from build123d import *

# Parameters (mm, degrees)
SKETCH_1_W          = 7.5
SKETCH_1_H          = 6
EXTRUDE_1_DEPTH     = 2
SKETCH_2_W          = 12.9
SKETCH_2_H          = 3.9
EXTRUDE_2_DEPTH     = 52
SKETCH_3_R          = 1.6
CUT_EXTRUDE_1_DEPTH = 356
SKETCH_4_W          = 7.5
SKETCH_4_H          = 1.05
CUT_EXTRUDE_2_DEPTH = 10


with BuildPart() as part:
    # 草图1 → 凸台-拉伸1 (new body)
    with BuildSketch(Plane.XY):
        with Locations((3.75, 0)):
            Rectangle(SKETCH_1_W, SKETCH_1_H)
    extrude(amount=EXTRUDE_1_DEPTH)

    # 草图2 → 凸台-拉伸2 (add)
    with BuildSketch(Plane.XY.offset(2)):
        Rectangle(SKETCH_2_W, SKETCH_2_H)
    extrude(amount=EXTRUDE_2_DEPTH)

    # 草图3 → 切除-拉伸1 (cut)
    with BuildSketch(Plane.XZ.offset(1.95)):
        with Locations((3.5, 37)):
            Circle(SKETCH_3_R)
        with Locations((3.5, 11)):
            Circle(SKETCH_3_R)
        with Locations((-3.5, 24)):
            Circle(SKETCH_3_R)
        with Locations((0, 50)):
            Circle(SKETCH_3_R)
    extrude(amount=-CUT_EXTRUDE_1_DEPTH, mode=Mode.SUBTRACT)

    # 草图4 → 切除-拉伸2 (cut)
    with BuildSketch(Plane.XY.offset(2)):
        with Locations((3.75, 2.475)):
            Rectangle(SKETCH_4_W, SKETCH_4_H)
    extrude(amount=-CUT_EXTRUDE_2_DEPTH, mode=Mode.SUBTRACT)


solid = part.part
The listing builds one solid part. Answer for the finished solid, in the listing's coordinates (mm). A direction names the side the tool comes from. Round coordinates to 2 decimals unless told otherwise and drop trailing zeros. Order: outer loops, then holes, each group sorted by start corner. A loop starts at its lowest first (then second) coordinate and runs counter-clockwise, first axis right, second up. Notation, with made-up numbers: (24, 67) -> (77, 67) arc R19 ccw to (77, 84) -> close; hole circle Ø6 at (4.5, -18.5). An arc over 180 degrees is marked (long way). Put each result on its own line as item: value.
Q1. Which of the six approach directions +Z, -Z, +X, -X, +Y, -Y give full straight-line access (tool end or side, diameter ignored) to faces 1 (the flat face through (-6.45, 0, 28)), 2 (the flat face through (6.45, 0, 28)), 3 (the flat face through (0, 0, 54)), 4 (the flat face through (-3, 0, 2)), 5 (the flat face through (0, -1.95, 28))?
Results list:
face 1: +Z, -Z, -X, +Y, -Y
face 2: +Z, +X, +Y, -Y
face 3: +Z, +X, -X, +Y, -Y
face 4: -Z, -X, +Y, -Y
face 5: +Z, +X, -X, -Y
Q2. Consider line 1 along Z through (x, y) = (3.5, -1.05); line 2 along Z through (x, y) = (4.25, -1.55); line 3 along Z through (x, y) = (-3.5, 0.2). Determine where each line is inside the solid, lowest interval first.
Results list:
line 1: 0 to 9.4, 12.6 to 35.4, 38.6 to 54
line 2: 0 to 9.59, 12.41 to 35.59, 38.41 to 54
line 3: 2 to 22.4, 25.6 to 54
Q3. Section B-B, the plane x = -2.5 is taken. Write down the section's boundary in (y, z).
Results list:
outline: (-1.95, 2) -> (1.95, 2) -> (1.95, 22.75) -> (-1.95, 22.75) -> close; (-1.95, 25.25) -> (1.95, 25.25) -> (1.95, 54) -> (-1.95, 54) -> close
Q4. Each of these flat-tipped pins is pushed along its axis until it touches: P1, Ø1, axis at x = -1.5, z = 37, coming from the -Y side; P2, Ø1, axis at y = -1.5, z = 1, coming from the -X side; P3, Ø1.2, axis at y = 0.5, z = 26, coming from the +X side. Where does it stop, or does it pass through?
Results list:
P1: y = -1.95
P2: x = 0
P3: x = 6.45
Q5. Determine the mould class of faces 6 (the flat face through (5.1, -2.2, 2)), 7 (the cylindrical face through (-3.708, -0.027, 25.586)), 8 (the flat face through (7.5, -1, 1)), 9 (the cylindrical face through (4.24, -0.03, 35.58)) for opening direction X: pulls with the +X half, pulls with the -X half, needs draft (parallel to the pull), parting line crosses it, or undercut.
Results list:
face 6: needs draft
face 7: undercut
face 8: pulls with the +X half
face 9: undercut
Q6. Section D-D, the plane x = 3.5 is taken. Write down the section's boundary in (y, z).
Results list:
outline: (-3, 0) -> (1.95, 0) -> (1.95, 9.4) -> (-1.95, 9.4) -> (-1.95, 2) -> (-3, 2) -> close; (-1.95, 12.6) -> (1.95, 12.6) -> (1.95, 35.4) -> (-1.95, 35.4) -> close; (-1.95, 38.6) -> (1.95, 38.6) -> (1.95, 54) -> (-1.95, 54) -> close
Q7. Section A-A, the plane y = 1.5 is taken. Write down the section's boundary in (x, z).
Results list:
outline: (-6.45, 2) -> (0, 2) -> (0, 0) -> (7.5, 0) -> (7.5, 2) -> (6.45, 2) -> (6.45, 54) -> (-6.45, 54) -> close; hole circle Ø3.2 at (-3.5, 24); hole circle Ø3.2 at (0, 50); hole circle Ø3.2 at (3.5, 11); hole circle Ø3.2 at (3.5, 37)
Q8. Section C-C, the plane z = 37 is taken. Write down the section's boundary in (x, y), and give its area (3 significant figures).
Results list:
outline: (-6.45, -1.95) -> (1.9, -1.95) -> (1.9, 1.95) -> (-6.45, 1.95) -> close; (5.1, -1.95) -> (6.45, -1.95) -> (6.45, 1.95) -> (5.1, 1.95) -> close
area: 37.8 mm^2
